Geometry: final body of the model. Coordinates: model frame, mm. A direction names the side the tool comes from. Round coordinates to 2 decimals unless told otherwise and drop trailing zeros. Order: outer loops, then holes, each group sorted by start corner. A loop starts at its lowest first (then second) coordinate and runs counter-clockwise, first axis right, second up. Notation, with made-up numbers: M 58.25,55 L 91.25,55 A18 ccw 91.25,62 Z; hole C 64.25,-18 d1. An arc over 180 degrees is marked long. Put each result on its own line as item: value. Start each with the question number.
1) Draft query along Z for faces 4 (the cylindrical face through (-12.13, 1.97, 6.99)), 5 (the cylindrical face through (-7.42, 1.97, 9.18)), 6 (the cylindrical face through (14, 2, 0)). Return one class per face: pulls with the +Z half, pulls with the -Z half, needs draft (parallel to the pull), parting line crosses it, or undercut.
2) Material intervals for probe 1 along X at (y, z) = (2.5, 12.5); probe 2 along X at (y, z) = (3.4, 12); probe 3 along X at (y, z) = (1.4, 0), sorted ascending. Write a range as [from, to].
3) Access query for faces 1 (the cylindrical face through (-4.29, 1.97, 11.07)), 2 (the cylindrical face through (11.07, 1.97, 4.29)), 3 (the cylindrical face through (-7.44, 1.97, -9.24)). Directions: +Z, -Z, +X, -X, +Y, -Y. A direction counts if a zero-diameter tool reaches every point of the face in a straight line with its end or side. Return the directions, or none.
4) Section B-B, the plane x = 0. Return loops of the section in (y, z) (3 decimals).
5) Section C-C, the plane x = -9.75. Return loops of the section in (y, z).
6) Section A-A, the plane z = 0. Return loops of the section in (x, y), then the cut area to 3 significant figures.
7) Section D-D, the plane z = -11. Return loops of the section in (x, y).
8) First-contact query: P1, Ø1.5, axis at y = 3, z = 8.5, coming from the -X side; P2, Ø0.7, axis at y = 3, z = -5.5, coming from the -X side; P3, Ø1, axis at y = 1, z = 3.5, coming from the -X side. Flat tips, straight axial feed; report the tip coordinate or a pass-through.
from build123d import *

# Parameters (mm, degrees)
EXTRUDE_1_DEPTH     = 4
CUT_EXTRUDE_1_DEPTH = 4


with BuildPart() as part:
    # 草图1 → 凸台-拉伸1 (new body)
    with BuildSketch(Plane(origin=(0, 0, 0), x_dir=(1, 0, 0), z_dir=(0, 1, 0))):
        with BuildLine():
            ThreePointArc((1.007141152, 13.96372682), (0, 14), (-1.007141152, 13.96372682))
            ThreePointArc((-1.007141152, 13.96372682), (-1.829065946, 11.692687307), (-2.012232645, 9.284445044))
            ThreePointArc((-2.012232645, 9.284445044), (-2.458780928, 9.17629535), (-2.899577934, 9.046681591))
            ThreePointArc((-2.899577934, 9.046681591), (-4.262326079, 11.04069722), (-6.109653587, 12.596512734))
            ThreePointArc((-6.109653587, 12.596512734), (-7, 12.124355653), (-7.854073233, 11.589371581))
            ThreePointArc((-7.854073233, 11.589371581), (-7.430361228, 9.211631273), (-6.384867111, 7.034448946))
            ThreePointArc((-6.384867111, 7.034448946), (-6.717514421, 6.717514421), (-7.034448946, 6.384867111))
            ThreePointArc((-7.034448946, 6.384867111), (-9.211631273, 7.430361228), (-11.589371581, 7.854073233))
            ThreePointArc((-11.589371581, 7.854073233), (-12.124355653, 7), (-12.596512734, 6.109653587))
            ThreePointArc((-12.596512734, 6.109653587), (-11.04069722, 4.262326079), (-9.046681591, 2.899577934))
            ThreePointArc((-9.046681591, 2.899577934), (-9.17629535, 2.458780928), (-9.284445044, 2.012232645))
            ThreePointArc((-9.284445044, 2.012232645), (-11.692687307, 1.829065946), (-13.96372682, 1.007141152))
            ThreePointArc((-13.96372682, 1.007141152), (-14, 0), (-13.96372682, -1.007141152))
            ThreePointArc((-13.96372682, -1.007141152), (-11.692687307, -1.829065946), (-9.284445044, -2.012232645))
            ThreePointArc((-9.284445044, -2.012232645), (-9.17629535, -2.458780928), (-9.046681591, -2.899577934))
            ThreePointArc((-9.046681591, -2.899577934), (-11.04069722, -4.262326079), (-12.596512734, -6.109653587))
            ThreePointArc((-12.596512734, -6.109653587), (-12.124355653, -7), (-11.589371581, -7.854073233))
            ThreePointArc((-11.589371581, -7.854073233), (-9.211631273, -7.430361228), (-7.034448946, -6.384867111))
            ThreePointArc((-7.034448946, -6.384867111), (-6.717514421, -6.717514421), (-6.384867111, -7.034448946))
            ThreePointArc((-6.384867111, -7.034448946), (-7.430361228, -9.211631273), (-7.854073233, -11.589371581))
            ThreePointArc((-7.854073233, -11.589371581), (-7, -12.124355653), (-6.109653587, -12.596512734))
            ThreePointArc((-6.109653587, -12.596512734), (-4.262326079, -11.04069722), (-2.899577934, -9.046681591))
            ThreePointArc((-2.899577934, -9.046681591), (-2.458780928, -9.17629535), (-2.012232645, -9.284445044))
            ThreePointArc((-2.012232645, -9.284445044), (-1.829065946, -11.692687307), (-1.007141152, -13.96372682))
            ThreePointArc((-1.007141152, -13.96372682), (0, -14), (1.007141152, -13.96372682))
            ThreePointArc((1.007141152, -13.96372682), (1.829065946, -11.692687307), (2.012232645, -9.284445044))
            ThreePointArc((2.012232645, -9.284445044), (2.458780928, -9.17629535), (2.899577934, -9.046681591))
            ThreePointArc((2.899577934, -9.046681591), (4.262326079, -11.04069722), (6.109653587, -12.596512734))
            ThreePointArc((6.109653587, -12.596512734), (7, -12.124355653), (7.854073233, -11.589371581))
            ThreePointArc((7.854073233, -11.589371581), (7.430361228, -9.211631273), (6.384867111, -7.034448946))
            ThreePointArc((6.384867111, -7.034448946), (6.717514421, -6.717514421), (7.034448946, -6.384867111))
            ThreePointArc((7.034448946, -6.384867111), (9.211631273, -7.430361228), (11.589371581, -7.854073233))
            ThreePointArc((11.589371581, -7.854073233), (12.124355653, -7), (12.596512734, -6.109653587))
            ThreePointArc((12.596512734, -6.109653587), (11.04069722, -4.262326079), (9.046681591, -2.899577934))
            ThreePointArc((9.046681591, -2.899577934), (9.17629535, -2.458780928), (9.284445044, -2.012232645))
            ThreePointArc((9.284445044, -2.012232645), (11.692687307, -1.829065946), (13.96372682, -1.007141152))
            ThreePointArc((13.96372682, -1.007141152), (14, 0), (13.96372682, 1.007141152))
            ThreePointArc((13.96372682, 1.007141152), (11.692687307, 1.829065946), (9.284445044, 2.012232645))
            ThreePointArc((9.284445044, 2.012232645), (9.17629535, 2.458780928), (9.046681591, 2.899577934))
            ThreePointArc((9.046681591, 2.899577934), (11.04069722, 4.262326079), (12.596512734, 6.109653587))
            ThreePointArc((12.596512734, 6.109653587), (12.124355653, 7), (11.589371581, 7.854073233))
            ThreePointArc((11.589371581, 7.854073233), (9.211631273, 7.430361228), (7.034448946, 6.384867111))
            ThreePointArc((7.034448946, 6.384867111), (6.717514421, 6.717514421), (6.384867111, 7.034448946))
            ThreePointArc((6.384867111, 7.034448946), (7.430361228, 9.211631273), (7.854073233, 11.589371581))
            ThreePointArc((7.854073233, 11.589371581), (7, 12.124355653), (6.109653587, 12.596512734))
            ThreePointArc((6.109653587, 12.596512734), (4.262326079, 11.04069722), (2.899577934, 9.046681591))
            ThreePointArc((2.899577934, 9.046681591), (2.458780928, 9.17629535), (2.012232645, 9.284445044))
            ThreePointArc((2.012232645, 9.284445044), (1.829065946, 11.692687307), (1.007141152, 13.96372682))
        make_face()
    extrude(amount=EXTRUDE_1_DEPTH)

    # 草图2 → 切除-拉伸1 (cut)
    with BuildSketch(Plane(origin=(0, 4, 0), x_dir=(1, 0, 0), z_dir=(0, 1, 0))):
        with BuildLine():
            Line((-1.095859036, 4.364526661), (-1.095859036, 6.645001166))
            Line((-1.095859036, 6.645001166), (1.095859036, 6.645001166))
            Line((1.095859036, 6.645001166), (1.095859036, 4.364526661))
            ThreePointArc((1.095859036, 4.364526661), (0, -4.5), (-1.095859036, 4.364526661))
        make_face()
    extrude(amount=-CUT_EXTRUDE_1_DEPTH, mode=Mode.SUBTRACT)


solid = part.part
Result sheet:
1. face 4: pulls with the +Z half
1. face 5: undercut
1. face 6: parting line crosses it
2. probe 1: x = [-6.3, -5.96], [-1.62, 1.62], [5.96, 6.3]
2. probe 2: x = [-7.21, -5.28], [-1.76, 1.76], [5.28, 7.21]
2. probe 3: x = [-14, -4.5], [4.5, 14]
3. face 1: +Z, +Y, -Y
3. face 2: +X, +Y, -Y
3. face 3: +Y, -Y
4. outline: M 0,-14 L 4,-14 L 4,-6.645 L 0,-6.645 Z; M 0,4.5 L 4,4.5 L 4,14 L 0,14 Z
5. outline: M 0,-7.59 L 4,-7.59 L 4,-3.29 L 0,-3.29 Z; M 0,-2.03 L 4,-2.03 L 4,2.03 L 0,2.03 Z; M 0,3.29 L 4,3.29 L 4,7.59 L 0,7.59 Z
6. outline: M -14,0 L -4.5,0 L -4.5,4 L -14,4 Z; M 4.5,0 L 14,0 L 14,4 L 4.5,4 Z
6. area: 76.0 mm2
7. outline: M -7.81,0 L -4.23,0 L -4.23,4 L -7.81,4 Z; M -1.95,0 L 1.95,0 L 1.95,4 L -1.95,4 Z; M 4.23,0 L 7.81,0 L 7.81,4 L 4.23,4 Z
8. P1: stops at x = -11.66
8. P2: stops at x = -12.43
8. P3: stops at x = -10.74
